```python
from build123d import *

# Parameters (mm, degrees)
SKETCH1_W           = 50
SKETCH1_H           = 80
BOSS_EXTRUDE1_DEPTH = 5
SKETCH2_W           = 13
SKETCH2_H           = 26
BOSS_EXTRUDE2_DEPTH = 2
SKETCH3_R           = 2.25
CUT_EXTRUDE1_DEPTH  = 48.68647607
FILLET1_R           = 10
FILLET2_R           = 6
FILLET3_R           = 1
CHAMFER1_SIZE       = 2.4


with BuildPart() as part:
    # Sketch1 → Boss-Extrude1 (new body)
    with BuildSketch(Plane(origin=(0, 0, 0), x_dir=(1, 0, 0), z_dir=(0, 1, 0))):
        Rectangle(SKETCH1_W, SKETCH1_H)
    extrude(amount=BOSS_EXTRUDE1_DEPTH)

    # Sketch2 → Boss-Extrude2 (add)
    with BuildSketch(Plane(origin=(0, 5, 0), x_dir=(1, 0, 0), z_dir=(0, 1, 0))):
        with Locations((0, 27)):
            Rectangle(SKETCH2_W, SKETCH2_H)
    extrude(amount=BOSS_EXTRUDE2_DEPTH)

    # Sketch3 → Cut-Extrude1 (cut, through all)
    with BuildSketch(Plane(origin=(0, 7, 0), x_dir=(1, 0, 0), z_dir=(0, 1, 0))):
        with Locations(Location((0, 35, 0), (0, 0, 270))):
            Circle(SKETCH3_R)
        with Locations(Location((0, 20, 0), (0, 0, 270))):
            Circle(SKETCH3_R)
    extrude(amount=-CUT_EXTRUDE1_DEPTH, mode=Mode.SUBTRACT)

    # Fillet1
    fillet1_edges = [part.edges().sort_by_distance(p)[0] for p in [
        (25, 2.5, 40),
        (-25, 2.5, 40),
        (-25, 2.5, -40),
        (25, 2.5, -40),
    ]]
    fillet(fillet1_edges, radius=FILLET1_R)

    # Fillet2
    # the kernel refuses this fillet: 6 mm, written as the material it adds along each edge
    with BuildSketch(Plane(origin=(6.5, 5, -14), x_dir=(1, 0, 0), z_dir=(0, 0, -1)), Plane(origin=(-6.5, 5, -40), x_dir=(-1, 0, 0), z_dir=(0, 0, 1))) as fillet2_piece_1:
        with BuildLine():
            CenterArc((4.472135955, -6), FILLET2_R, 90, 48.189685104)
            Line((0, -2), (-0.089442719, -1.92))
            ThreePointArc((-0.089442719, -1.92), (-0.12, -1), (-0.12, 0))
            Line((-0.12, 0), (0, 0.12))
            Line((0, 0.12), (4.472135955, 0.12))
            Line((4.472135955, 0.12), (4.472135955, 0))
        make_face()
    extrude(amount=26)
    with BuildSketch(Plane(origin=(-6.5, 5, -14), x_dir=(0, 0, 1), z_dir=(1, 0, 0))) as fillet2_piece_2:
        with BuildLine():
            CenterArc((4.472135955, -6), FILLET2_R, 90, 48.189685104)
            Line((0, -2), (-0.089442719, -1.92))
            ThreePointArc((-0.089442719, -1.92), (-0.12, -1), (-0.12, 0))
            Line((-0.12, 0), (0, 0.12))
            Line((0, 0.12), (4.472135955, 0.12))
            Line((4.472135955, 0.12), (4.472135955, 0))
        make_face()
    extrude(amount=13)
    with BuildSketch(Plane(origin=(-6.5, 5, -14), x_dir=(0, 0, 1), z_dir=(1, 0, 0))) as fillet2_piece_3a_section:
        with BuildLine():
            CenterArc((4.472135955, -6), FILLET2_R, 90, 48.189685104)
            Line((0, -2), (-0.089442719, -1.92))
            ThreePointArc((-0.089442719, -1.92), (-0.12, -1), (-0.12, 0))
            Line((-0.12, 0), (0, 0.12))
            Line((0, 0.12), (4.472135955, 0.12))
            Line((4.472135955, 0.12), (4.472135955, 0))
        make_face()
    fillet2_piece_3a = extrude(amount=24.180339887, mode=Mode.PRIVATE)
    fillet2_piece_3a = split(fillet2_piece_3a, bisect_by=Plane(origin=(6.5, 5.502082099, -12.82079949), z_dir=(1, 0, 0)), keep=Keep.TOP, mode=Mode.PRIVATE)
    with BuildSketch(Plane(origin=(6.5, 5, -2.819660113), x_dir=(1, 0, 0), z_dir=(0, 0, -1))) as fillet2_piece_3b_section:
        with BuildLine():
            CenterArc((4.472135955, -6), FILLET2_R, 90, 48.189685104)
            Line((0, -2), (-0.089442719, -1.92))
            ThreePointArc((-0.089442719, -1.92), (-0.12, -1), (-0.12, 0))
            Line((-0.12, 0), (0, 0.12))
            Line((0, 0.12), (4.472135955, 0.12))
            Line((4.472135955, 0.12), (4.472135955, 0))
        make_face()
    fillet2_piece_3b = extrude(amount=37.180339887, mode=Mode.PRIVATE)
    fillet2_piece_3b = split(fillet2_piece_3b, bisect_by=Plane(origin=(7.67920051, 5.502082099, -14), z_dir=(0, 0, 1)), keep=Keep.TOP, mode=Mode.PRIVATE)
    fillet2_piece_3 = fillet2_piece_3a & fillet2_piece_3b
    add(fillet2_piece_3)
    with BuildSketch(Plane(origin=(-6.5, 5, -40), x_dir=(-1, 0, 0), z_dir=(0, 0, 1))) as fillet2_piece_4a_section:
        with BuildLine():
            CenterArc((4.472135955, -6), FILLET2_R, 90, 48.189685104)
            Line((0, -2), (-0.089442719, -1.92))
            ThreePointArc((-0.089442719, -1.92), (-0.12, -1), (-0.12, 0))
            Line((-0.12, 0), (0, 0.12))
            Line((0, 0.12), (4.472135955, 0.12))
            Line((4.472135955, 0.12), (4.472135955, 0))
        make_face()
    fillet2_piece_4a = extrude(amount=37.180339887, mode=Mode.PRIVATE)
    fillet2_piece_4a = split(fillet2_piece_4a, bisect_by=Plane(origin=(-7.67920051, 5.502082099, -14), z_dir=(0, 0, 1)), keep=Keep.TOP, mode=Mode.PRIVATE)
    with BuildSketch(Plane(origin=(-17.680339887, 5, -14), x_dir=(0, 0, 1), z_dir=(1, 0, 0))) as fillet2_piece_4b_section:
        with BuildLine():
            CenterArc((4.472135955, -6), FILLET2_R, 90, 48.189685104)
            Line((0, -2), (-0.089442719, -1.92))
            ThreePointArc((-0.089442719, -1.92), (-0.12, -1), (-0.12, 0))
            Line((-0.12, 0), (0, 0.12))
            Line((0, 0.12), (4.472135955, 0.12))
            Line((4.472135955, 0.12), (4.472135955, 0))
        make_face()
    fillet2_piece_4b = extrude(amount=24.180339887, mode=Mode.PRIVATE)
    fillet2_piece_4b = split(fillet2_piece_4b, bisect_by=Plane(origin=(-6.5, 5.502082099, -12.82079949), z_dir=(-1, 0, 0)), keep=Keep.TOP, mode=Mode.PRIVATE)
    fillet2_piece_4 = fillet2_piece_4a & fillet2_piece_4b
    add(fillet2_piece_4)

    # Fillet3
    fillet3_edges = [part.edges().sort_by_distance(p)[0] for p in [
        (12.986067978, 5, -40),
        (25, 5, 0),
        (-25, 5, 0),
        (0, 5, 40),
        (-22.071067812, 5, -37.071067812),
        (-22.071067812, 5, 37.071067812),
        (22.071067812, 5, 37.071067812),
        (22.071067812, 5, -37.071067812),
        (-12.986067977, 5, -40),
        (8.522646212, 5.522774425, -40),
        (-8.522646212, 5.522774425, -40),
    ]]
    fillet(fillet3_edges, radius=FILLET3_R)

    # Chamfer1
    chamfer1_edges = [part.edges().sort_by_distance(p)[0] for p in [
        (0, 0, -37.25),
        (0, 0, -22.25),
    ]]
    chamfer(chamfer1_edges, length=CHAMFER1_SIZE)


solid = part.part
```
Verification items for the finished model (mm, model axes). Give positions to 0.01 mm unless a question says otherwise; leave off trailing zeros. Order: outer loops, then holes, each group sorted by start corner. A loop starts at its lowest first (then second) coordinate and runs counter-clockwise, first axis right, second up. Notation, with made-up numbers: M -20.75,19 L 29.25,19 A12 cw 29.25,26 Z; hole C 49.5,1.25 d7. An arc over 180 degrees is marked long. Return JSON: item names as keys, results as strings. Group by question number.
1) Section check C-C on y = 1.5. Record the cut outline in (x, z).
2) Section check D-D on x = 14. Record the cut outline in (y, z), and give its area (3 significant figures).
3) Scan lines: line 1 (X direction, y = 3.7, z = -35); line 2 (Y direction, x = -8, z = 17.5); line 3 (X direction, y = 4.8, z = -35). Record each from-to range of solid material in increasing order.
4) Go/stop test with flat-tipped pins: pin 1 Ø1.5 at (x, z) = (-12.5, 3) entering from -Y; pin 2 Ø5 at (x, z) = (0, -35) entering from -Y; pin 3 Ø6 at (x, z) = (0, -20) entering from -Y; pin 4 Ø2 at (x, z) = (7.5, 8.5) entering from +Y. Record where each tip stops, or that it passes through.
5) Section check A-A on z = -20. Record the cut outline in (x, y).
6) Section check B-B on x = 0. Record the cut outline in (y, z).
7) Mould release check, pull along X, two halves, no side actions. Record for faces 1 (the face through (0, 3, -40)), 2 (the face through (-0.86, 4.73, -32.92)), 3 (the face through (21.99, 2.03, 37.15)): pulls with the +X half, pulls with the -X half, needs draft (parallel to the pull), parting line crosses it, or undercut.
Answer block:
{
 "1": {"outline": "M -25,-30 A10 ccw -15,-40 L 15,-40 A10 ccw 25,-30 L 25,30 A10 ccw 15,40 L -15,40 A10 ccw -25,30 Z; hole C 0,-35 d6.3; hole C 0,-20 d6.3"},
 "2": {"outline": "M 0,-40 L 4,-40 A1 ccw 5,-39 L 5,39 A1 ccw 4,40 L 0,40 Z", "area": "400 mm^2"},
 "3": {"line 1": "x = -23.66 to -2.25, 2.25 to 23.66", "line 2": "y = 0 to 5", "line 3": "x = -23.2 to -2.25, 2.25 to 23.2"},
 "4": {"pin 1": "stops at y = 0", "pin 2": "stops at y = 2.15", "pin 3": "stops at y = 1.65", "pin 4": "stops at y = 5"},
 "5": {"outline": "M -25,0 L -4.65,0 L -2.25,2.4 L -2.25,7 L -6.5,7 A6 cw -10.97,5 L -24,5 A1 ccw -25,4 Z; M 2.25,2.4 L 4.65,0 L 25,0 L 25,4 A1 ccw 24,5 L 10.97,5 A6 cw 6.5,7 L 2.25,7 Z"},
 "6": {"outline": "M 0,-40 L 7,-40 L 7,-37.25 L 2.4,-37.25 L 0,-39.65 Z; M 0,-30.35 L 2.4,-32.75 L 7,-32.75 L 7,-22.25 L 2.4,-22.25 L 0,-24.65 Z; M 0,-15.35 L 2.4,-17.75 L 7,-17.75 L 7,-14 A6 cw 5,-9.53 L 5,39 A1 ccw 4,40 L 0,40 Z"},
 "7": {"face 1": "needs draft", "face 2": "undercut", "face 3": "pulls with the +X half"}
}
